Verification items for this drawing (mm, ordinates from the low corner). A direction names the side the tool comes from. Round coordinates to 2 decimals unless told otherwise and drop trailing zeros. Write each loop counter-clockwise with the first axis right and the second up, starting at its lowest first coordinate (ties: lowest second). Pieces come first, ordered by that corner, then holes.
Item 1: Scan lines: probe 1 along Y at (x, z) = (47.5, 3.5); probe 2 along X at (y, z) = (93, 5.75); probe 3 along X at (y, z) = (78, 7.75) (1 decimal). Record each from-to range of solid material in increasing order.
Item 2: Cross-section at D-D (x = 69.5). Enter the section's corners in (y, z).
Item 3: Cross-section at B-B (x = 47.5). Enter the section's corners in (y, z).
Item 4: Cross-section at C-C (z = 4.75). Enter the section's corners in (x, y).
Item 5: Access from +Z, -Z, +X, -X, +Y, -Y to the whole of each face (thin tool, end or side, straight path). Record for the marked faces 4 and 5.
Item 6: Depth check by flat-ended pin: P1, Ø5, axis at x = 74.35, y = 77.5, coming from the +Z side; P2, Ø3, axis at x = 12, z = 6.5, coming from the -Y side; P3, Ø3, axis at y = 3, z = 6.5, coming from the +X side; P4, Ø5, axis at y = 5, z = 4, coming from the -X side. Enter the tip coordinate at first touch or a pass-through.
Item 7: Cross-section at A-A (y = 93). Enter the section's corners in (x, z).
Item 8: Draft check along X on the marked faces 1, 2 and 3. Enter one of: pulls with the +X half, pulls with the -X half, needs draft (parallel to the pull), parting line crosses it, or undercut.
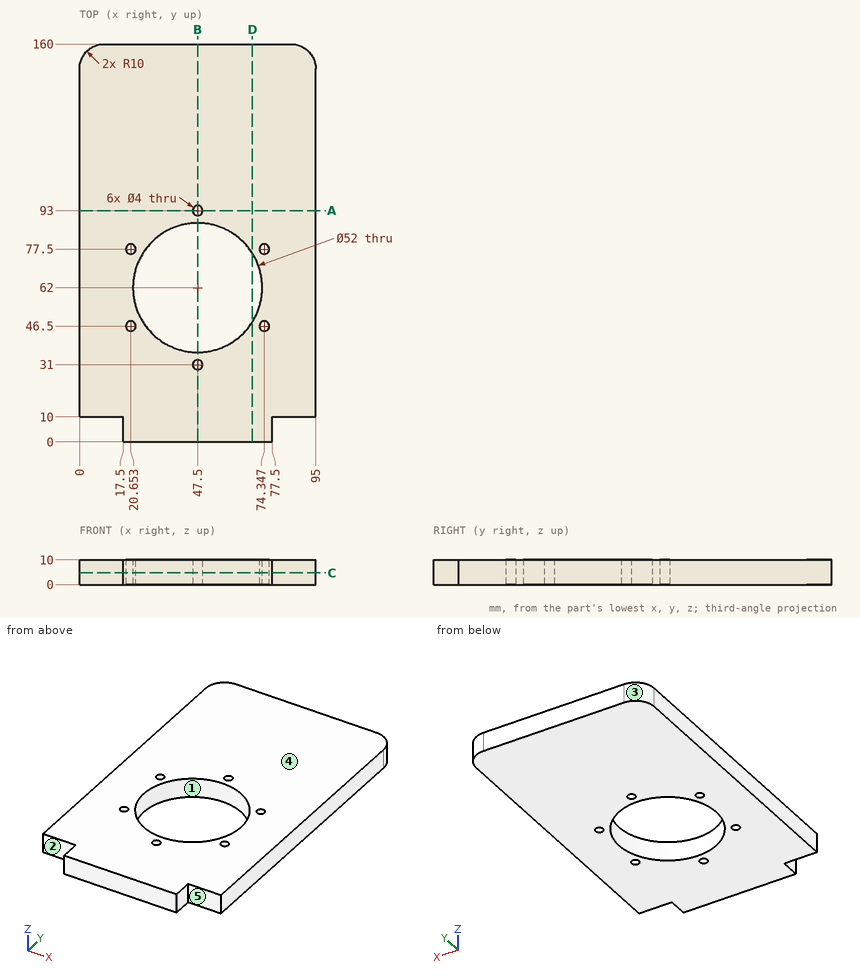
Resolved:
1. probe 1: y = 0 to 29, 33 to 36, 88 to 91, 95 to 160
1. probe 2: x = 0 to 45.5, 49.5 to 95
1. probe 3: x = 0 to 18.7, 22.6 to 27, 68 to 72.4, 76.3 to 95
2. outline: (0, 0) - (48.14, 0) - (48.14, 10) - (0, 10) - close; (75.86, 0) - (160, 0) - (160, 10) - (75.86, 10) - close
3. outline: (0, 0) - (29, 0) - (29, 10) - (0, 10) - close; (33, 0) - (36, 0) - (36, 10) - (33, 10) - close; (88, 0) - (91, 0) - (91, 10) - (88, 10) - close; (95, 0) - (160, 0) - (160, 10) - (95, 10) - close
4. outline: (0, 10) - (17.5, 10) - (17.5, 0) - (77.5, 0) - (77.5, 10) - (95, 10) - (95, 150) arc R10 ccw to (85, 160) - (10, 160) arc R10 ccw to (0, 150) - close; hole circle Ø4 at (20.65, 46.5); hole circle Ø4 at (20.65, 77.5); hole circle Ø52 at (47.5, 62); hole circle Ø4 at (47.5, 31); hole circle Ø4 at (47.5, 93); hole circle Ø4 at (74.35, 46.5); hole circle Ø4 at (74.35, 77.5)
5. face 4: +Z, +X, -X, +Y, -Y
5. face 5: +Z, -Z, +X, -Y
6. P1: stops at z = 10
6. P2: stops at y = 10
6. P3: stops at x = 77.5
6. P4: stops at x = 17.5
7. outline: (0, 0) - (45.5, 0) - (45.5, 10) - (0, 10) - close; (49.5, 0) - (95, 0) - (95, 10) - (49.5, 10) - close
8. face 1: undercut
8. face 2: needs draft
8. face 3: pulls with the -X half
